from build123d import *

# Parameters (mm, degrees)
BOSS_EXTRUDE1_DEPTH = 8
FILLET1_R           = 0.5
SKETCH2_R           = 1.5
CUT_EXTRUDE1_DEPTH  = 3.682236538


with BuildPart() as part:
    # Sketch1 → Boss-Extrude1 (new body)
    with BuildSketch(Plane.XY):
        with BuildLine():
            Line((-4, -6.92820323), (-4, -9.92820323))
            Line((-4, -9.92820323), (4, -9.92820323))
            Line((4, -9.92820323), (4, -6.92820323))
            ThreePointArc((4, -6.92820323), (0, -8), (-4, -6.92820323))
        make_face()
    extrude(amount=BOSS_EXTRUDE1_DEPTH)

    # Fillet1
    fillet1_edges = [part.edges().sort_by_distance(p)[0] for p in [
        (4, -6.92820323, 4),
        (-4, -6.92820323, 4),
    ]]
    fillet(fillet1_edges, radius=FILLET1_R)

    # Sketch2 → Cut-Extrude1 (cut, through all)
    with BuildSketch(Plane.XZ.offset(9.92820323)):
        with Locations((0, 4)):
            Circle(SKETCH2_R)
    extrude(amount=-CUT_EXTRUDE1_DEPTH, mode=Mode.SUBTRACT)


solid = part.part
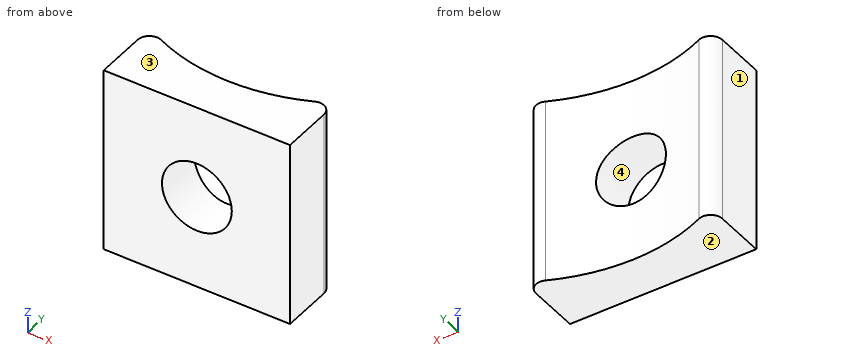
Geometry: final body of the model. Coordinates: model frame, mm. Face numbers are marked on the shaded views. Coordinates: 2 decimals unless noted, no trailing zeros. Loops run counter-clockwise (first coordinate to the right, second up) from the corner with the lowest first, then second, coordinate; pieces in that order, holes last. Notation, with made-up numbers: M 88,-16.5 L 102,-16.5 A6 ccw 102,-10.5 Z; hole C -8,33 d1. An arc over 180 degrees is marked long. One line per item, written item: value. Start each with the question number.
1) Cut plane B-B (z = 4). Return loops of the section in (x, y), then the cut area to 3 significant figures.
2) Material intervals for L1, parallel to Z at x = 0, y = -9.25; L2, parallel to X at y = -8.8, z = 4; L3, parallel to Y at x = 0, z = 6, sorted ascending. Write a range as from..to.
3) Cut plane C-C (y = -9). Return loops of the section in (x, z).
4) Draft query along Z for the marked faces 1, 2, 3 and 4. Return one class per face: released by +Z, released by -Z, zero draft, split by the parting line, or undercut.
5) Cut plane A-A (x = 0). Return loops of the section in (y, z), then the cut area to 3 significant figures.
6) Cut plane D-D (z = 1). Return loops of the section in (x, y), then the cut area to 3 significant figures.
Evaluation:
1. outline: M -4,-9.93 L -1.5,-9.93 L -1.5,-7.86 A8 cw -3.29,-7.29 A0.5 ccw -4,-7.75 Z; M 1.5,-9.93 L 4,-9.93 L 4,-7.75 A0.5 ccw 3.29,-7.29 A8 cw 1.5,-7.86 Z
1. area: 12.0 mm^2
2. L1: 0..2.5, 5.5..8
2. L2: -4..-1.5, 1.5..4
2. L3: -9.93..-8
3. outline: M -4,0 L 4,0 L 4,8 L -4,8 Z; hole C 0,4 d3
4. face 1: zero draft
4. face 2: released by -Z
4. face 3: released by +Z
4. face 4: undercut
5. outline: M -9.93,0 L -8,0 L -8,2.5 L -9.93,2.5 Z; M -9.93,5.5 L -8,5.5 L -8,8 L -9.93,8 Z
5. area: 9.64 mm^2
6. outline: M -4,-9.93 L 4,-9.93 L 4,-7.75 A0.5 ccw 3.29,-7.29 A8 cw -3.29,-7.29 A0.5 ccw -4,-7.75 Z
6. area: 17.9 mm^2
